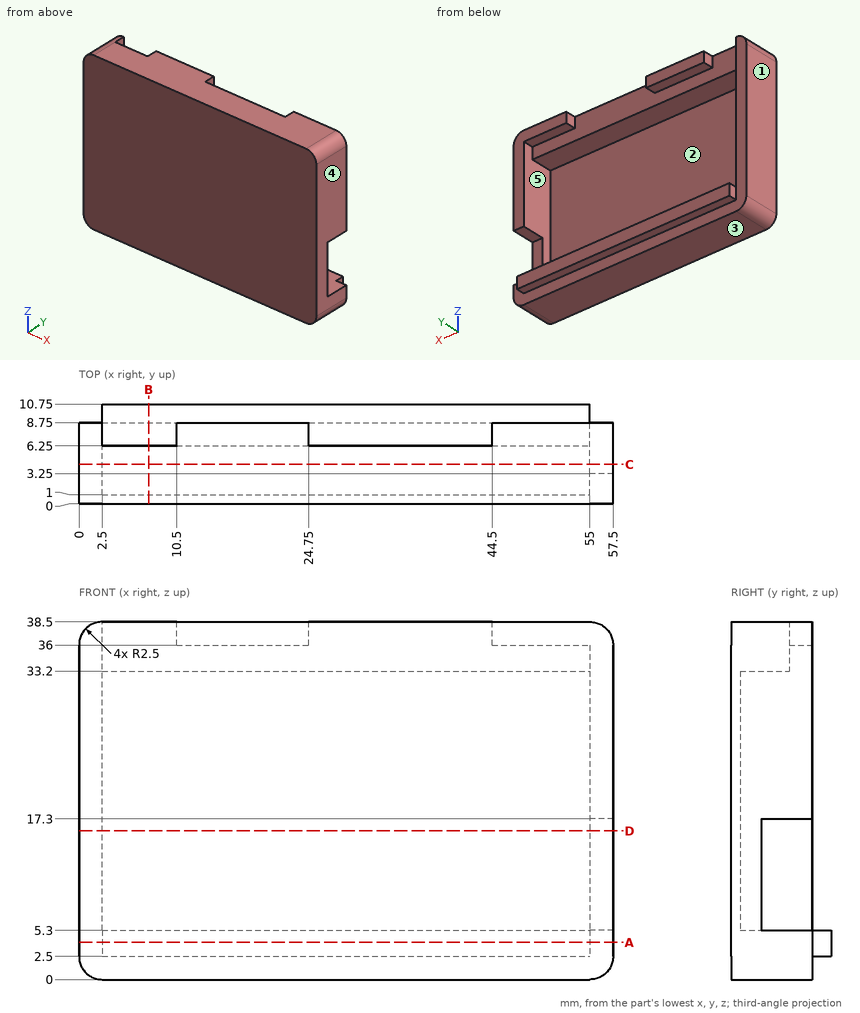
Design review of the part shown in the three views and the two pictorial views. Dimensions are in mm from the part's minimum x, y and z. A direction names the side the tool comes from. Coordinates: 2 decimals unless noted, no trailing zeros. Write each loop counter-clockwise with the first axis right and the second up, starting at its lowest first coordinate (ties: lowest second). Pieces come first, ordered by that corner, then holes. Notation, with made-up numbers: (40, 6) - (84, 6) arc R36 ccw to (84, 40) - close; hole circle Ø3 at (-16.75, 25.25). An arc over 180 degrees is marked (long way). Write item = value, one per line.
(1) Consider section B-B, the plane x = 7.5. Give the boundary of the cut face in (y, z).
Result sheet:
outline = (0, 0) - (8.75, 0) - (8.75, 2.5) - (10.75, 2.5) - (10.75, 5.3) - (1, 5.3) - (1, 33.2) - (6.25, 33.2) - (6.25, 38.5) - (0, 38.5) - close
(2) For line 1 (Z direction, x = 33, y = 6); line 2 (X direction, y = 2.5, z = 21); line 3 (Z direction, x = 15, y = 7.75), list the stretches that pass through material, from the lowest coordinate up. Write a range as [from, to].
Result sheet:
line_1 = [0, 5.3], [33.2, 38.5]
line_2 = [0, 2.5], [55, 57.5]
line_3 = [0, 5.3], [36, 38.5]
(3) Consider section A-A, the plane z = 4. Give the boundary of the cut face in (x, y), then the cut area to 3 significant figures.
Result sheet:
outline = (0, 0) - (57.5, 0) - (57.5, 8.75) - (55, 8.75) - (55, 10.75) - (2.5, 10.75) - (2.5, 8.75) - (0, 8.75) - close
area = 608 mm^2
(4) For P1, Ø2, axis at y = 7.5, z = 38, coming from the +X side; P2, Ø1, axis at y = 8, z = 5.5, coming from the +X side; P3, Ø0.6, axis at y = 10, z = 4, coming from the -X side; P4, Ø0.8, axis at x = 56.5, z = 12, coming from the +Y side, all flat-tipped, find the tip position at first contact; note any pin that passes through.
Result sheet:
P1 = 57.29
P2 = 57.5
P3 = 2.5
P4 = 3.25
(5) Mouldability with a two-part tool opening along Z and no side actions: class the marked faces 1, 2 and 3 as pulls with the +Z half, pulls with the -Z half, needs draft (parallel to the pull), parting line crosses it, or undercut.
Result sheet:
face_1 = needs draft
face_2 = undercut
face_3 = pulls with the -Z half
(6) Consider section D-D, the plane z = 16. Give the boundary of the cut face in (x, y), then the cut area to 3 significant figures.
Result sheet:
outline = (0, 0) - (57.5, 0) - (57.5, 3.25) - (55, 3.25) - (55, 1) - (2.5, 1) - (2.5, 8.75) - (0, 8.75) - close
area = 82.5 mm^2
(7) Consider section C-C, the plane y = 4.25. Give the boundary of the cut face in (x, z).
Result sheet:
outline = (0, 2.5) arc R2.5 ccw to (2.5, 0) - (55, 0) arc R2.5 ccw to (57.5, 2.5) - (57.5, 5.3) - (2.5, 5.3) - (2.5, 33.2) - (55, 33.2) - (55, 17.3) - (57.5, 17.3) - (57.5, 36) arc R2.5 ccw to (55, 38.5) - (2.5, 38.5) arc R2.5 ccw to (0, 36) - close
(8) Machinability: for the marked faces 4 and 5, which of the approach directions +Z, -Z, +X, -X, +Y, -Y give a long, thin tool a straight path to every point of the face, cutting with its end or side? Answer none if there is none.
Result sheet:
face_4 = +Z, -Z, +X, +Y, -Y
face_5 = +Y
